Verification items for the finished model (mm, model axes). Face numbers are marked on the shaded views. A direction names the side the tool comes from. Round coordinates to 2 decimals unless told otherwise and drop trailing zeros. Write each loop counter-clockwise with the first axis right and the second up, starting at its lowest first coordinate (ties: lowest second). Pieces come first, ordered by that corner, then holes. Notation, with made-up numbers: (6, 80) - (32, 80) arc R14 cw to (32, 91) - close; hole circle Ø3 at (66.5, 35.25). An arc over 180 degrees is marked (long way). Answer as a JSON object with one key per item and string values. Group by question number.
1) Section check A-A (z = 14). Enter the section's corners in (x, y).
2) Set-up check for the marked faces 1 and 2: record each of +Z, -Z, +X, -X, +Y, -Y from which the full face is reachable in a straight line by a thin tool's end or side.
3) Thickness scan on line 1 (X direction, y = 1.5, z = 44.5); line 2 (Y direction, x = 18.5, z = 18.5); line 3 (Y direction, x = 14, z = 9). Record the ranges inside material, lowest first.
4) Section check D-D (z = 37). Enter the section's corners in (x, y).
5) Section check C-C (y = 2.5). Enter the section's corners in (x, z), then the cut area to 3 significant figures.
6) Go/stop test with flat-tipped pins: pin 1 Ø1.5 at (y, z) = (5, 16.5) entering from -X; pin 2 Ø4 at (y, z) = (4, 22.5) entering from +X; pin 3 Ø4 at (x, z) = (43, 23) entering from -Y. Record where each tip stops, or that it passes through.
7) Section check B-B (x = 27). Enter the section's corners in (y, z), then the cut area to 3 significant figures.
```python
from build123d import *

# Parameters (mm, degrees)
Y_KSEKLIK_EKSTR_ZYON1_DEPTH = 46
RADYUS1_DEPTH               = 49


with BuildPart() as part:
    # Çizim1 → Yükseklik-Ekstrüzyon1 (new body)
    with BuildSketch(Plane.XY):
        Polygon((0, 0), (0, 13), (49, 13), (49, 10), (3, 10), (3, 0), align=None)
    extrude(amount=Y_KSEKLIK_EKSTR_ZYON1_DEPTH)

    # Radyus1: read off the stored shape, not the designer's step
    # Radyus1 outline → Radyus1 (cut)
    with BuildSketch(Plane.YZ):
        with BuildLine():
            Line((0, 0), (13, 0))
            Line((13, 0), (13, 15.716233646))
            ThreePointArc((13, 15.716233646), (9.328828006, 5.518194618), (0, 0))
        make_face()
    extrude(amount=RADYUS1_DEPTH, mode=Mode.SUBTRACT)


solid = part.part
```
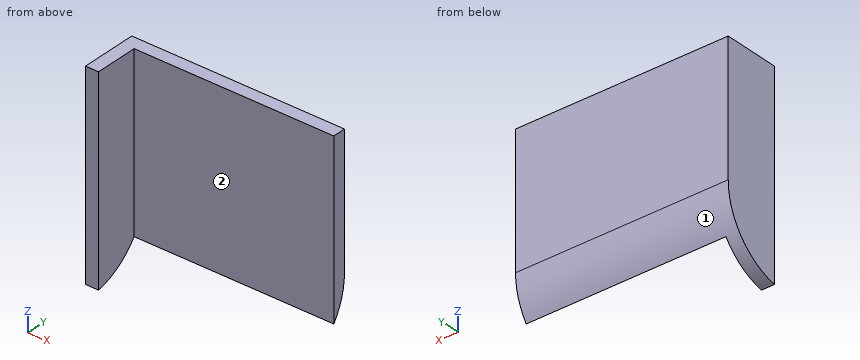
Returned:
{
 "1": {"outline": "(0, 0) - (3, 0) - (3, 10) - (49, 10) - (49, 12.91) - (0, 12.91) - close"},
 "2": {"face 1": "-Z, +X, -X, +Y", "face 2": "+Z, -Z, +X, -Y"},
 "3": {"line 1": "0 to 3", "line 2": "10 to 13", "line 3": "10 to 11.52"},
 "4": {"outline": "(0, 0) - (3, 0) - (3, 10) - (49, 10) - (49, 13) - (0, 13) - close"},
 "5": {"outline": "(0, 0.69) - (3, 0.69) - (3, 46) - (0, 46) - close", "area": "136 mm2"},
 "6": {"pin 1": "x = 0", "pin 2": "x = 3", "pin 3": "y = 10"},
 "7": {"outline": "(10, 6.39) arc R16 ccw to (13, 15.72) - (13, 46) - (10, 46) - close", "area": "110 mm2"}
}
